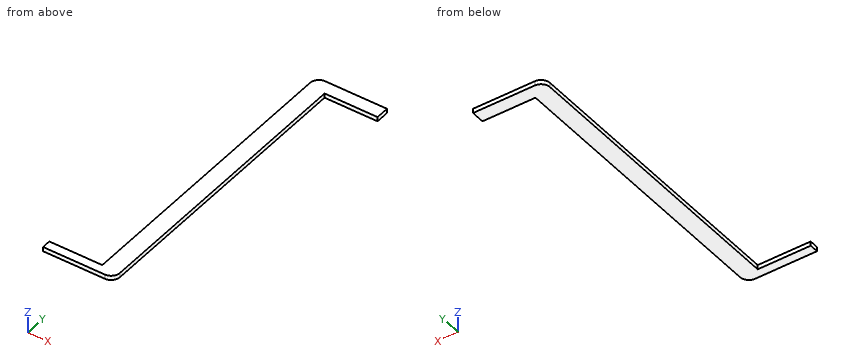
Solid Edge part; units mm, degrees
sketch "Sketch1" plane through (0, 0, 0) normal (0, 0, 1) x (1, 0, 0)
  line L0 (14, 35) -> (14, 32)
  line L1 (14, 32) -> (2, 32)
  line L2 (2, 32) -> (2, -33)
  arc A0 (2, -33) -> (0, -35) centre (0, -33) cw
  line L3 (0, -35) -> (-14, -35)
  line L4 (-14, -35) -> (-14, -33)
  line L5 (-14, -33) -> (-2, -33)
  line L6 (-2, -33) -> (-2, 33)
  arc A1 (-2, 33) -> (0, 35) centre (0, 33) cw
  line L7 (14, 35) -> (0, 35)
  dimension "D1" = 14
  dimension "D2" = 14
  dimension "D3" = 14
  dimension "D4" = 2
  dimension "D5" = 2
  dimension "D6" = 2
extrude "Ajout_matière_1" add sketch "Sketch1" along normal blind 1
properties material "Acier S235"
Read the model definition and answer for the solid it produces. Units are mm, in the model's axes. Coordinates: 2 decimals unless noted, no trailing zeros. Order: outer loops, then holes, each group sorted by start corner. A loop starts at its lowest first (then second) coordinate and runs counter-clockwise, first axis right, second up. Notation, with made-up numbers: (42, -5.75) - (70, -5.75) arc R17 cw to (70, 1.25) - close; hole circle Ø11 at (54, -9). An arc over 180 degrees is marked (long way). Answer as a JSON object with one key per item and string values. Group by question number.
Item 1: Section A-A (z = 0.15) is taken. Give the vertices of the cut face in (x, y), plus the area to 3 significant figures.
Item 2: Section B-B (y = 2) is taken. Give the vertices of the cut face in (x, z).
Item 3: Section C-C (x = 10.5) is taken. Give the vertices of the cut face in (y, z).
Item 4: Consider probe 1 along X at (y, z) = (12.5, 0.35); probe 2 along Y at (x, z) = (-8.5, 0.9); probe 3 along Y at (x, z) = (6.75, 0.35). Determine where each line is inside the solid, lowest interval first. Write a range as from..to.
Item 5: Flat-ended cylindrical pins translate along their axes: P1, Ø0.5, axis at y = -3.5, z = 0.5, coming from the +X side; P2, Ø6, axis at x = 6, y = 20.5, coming from the +Z side. Find the tip coordinate at first contact, or state that the pin passes through.
Results are:
{
 "1": {"outline": "(-14, -35) - (0, -35) arc R2 ccw to (2, -33) - (2, 32) - (14, 32) - (14, 35) - (0, 35) arc R2 ccw to (-2, 33) - (-2, -33) - (-14, -33) - close", "area": "338 mm^2"},
 "2": {"outline": "(-2, 0) - (2, 0) - (2, 1) - (-2, 1) - close"},
 "3": {"outline": "(32, 0) - (35, 0) - (35, 1) - (32, 1) - close"},
 "4": {"probe 1": "x = -2..2", "probe 2": "y = -35..-33", "probe 3": "y = 32..35"},
 "5": {"P1": "stops at x = 2", "P2": "passes through"}
}
